from build123d import *

# Parameters (mm, degrees)
SKETCH_1_W          = 80
SKETCH_1_H          = 80
EXTRUDE_1_DEPTH     = 2
CUT_EXTRUDE_1_DEPTH = 10


with BuildPart() as part:
    # ｽｹｯﾁ1 → ﾎﾞｽ - 押し出し1 (new body)
    with BuildSketch(Plane.XY):
        Rectangle(SKETCH_1_W, SKETCH_1_H)
    extrude(amount=EXTRUDE_1_DEPTH)

    # ｽｹｯﾁ2 → ｶｯﾄ - 押し出し1 (cut)
    with BuildSketch(Plane.XY.offset(2)):
        with BuildLine():
            ThreePointArc((29.5, -25), (26.318019485, -26.318019485), (25, -29.5))
            Line((25, -29.5), (29.5, -29.5))
            Line((29.5, -29.5), (29.5, -25))
        make_face()
        with BuildLine():
            Line((29.5, -29.5), (25, -29.5))
            ThreePointArc((25, -29.5), (29.5, -34), (34, -29.5))
            ThreePointArc((34, -29.5), (32.681980515, -26.318019485), (29.5, -25))
            Line((29.5, -25), (29.5, -29.5))
        make_face()
        with BuildLine():
            ThreePointArc((21.99, -17.49), (18.808019485, -18.808019485), (17.49, -21.99))
            Line((17.49, -21.99), (21.99, -21.99))
            Line((21.99, -21.99), (21.99, -17.49))
        make_face()
        with BuildLine():
            Line((21.99, -21.99), (17.49, -21.99))
            ThreePointArc((17.49, -21.99), (21.99, -26.49), (26.49, -21.99))
            ThreePointArc((26.49, -21.99), (25.171980515, -18.808019485), (21.99, -17.49))
            Line((21.99, -17.49), (21.99, -21.99))
        make_face()
        with BuildLine():
            ThreePointArc((25, 29.5), (26.318019485, 26.318019485), (29.5, 25))
            Line((29.5, 25), (29.5, 29.5))
            Line((29.5, 29.5), (25, 29.5))
        make_face()
        with BuildLine():
            Line((29.5, 29.5), (29.5, 25))
            ThreePointArc((29.5, 25), (32.681980515, 26.318019485), (34, 29.5))
            ThreePointArc((34, 29.5), (29.5, 34), (25, 29.5))
            Line((25, 29.5), (29.5, 29.5))
        make_face()
        with BuildLine():
            ThreePointArc((17.49, 21.99), (18.808019485, 18.808019485), (21.99, 17.49))
            Line((21.99, 17.49), (21.99, 21.99))
            Line((21.99, 21.99), (17.49, 21.99))
        make_face()
        with BuildLine():
            Line((21.99, 21.99), (21.99, 17.49))
            ThreePointArc((21.99, 17.49), (25.171980515, 18.808019485), (26.49, 21.99))
            ThreePointArc((26.49, 21.99), (21.99, 26.49), (17.49, 21.99))
            Line((17.49, 21.99), (21.99, 21.99))
        make_face()
        with BuildLine():
            ThreePointArc((-21.99, -17.49), (-25.171980515, -25.171980515), (-17.49, -21.99))
            Line((-17.49, -21.99), (-21.99, -21.99))
            Line((-21.99, -21.99), (-21.99, -17.49))
        make_face()
        with BuildLine():
            Line((-21.99, -21.99), (-17.49, -21.99))
            ThreePointArc((-17.49, -21.99), (-18.808019485, -18.808019485), (-21.99, -17.49))
            Line((-21.99, -17.49), (-21.99, -21.99))
        make_face()
        with BuildLine():
            ThreePointArc((-29.5, -25), (-32.681980515, -32.681980515), (-25, -29.5))
            Line((-25, -29.5), (-29.5, -29.5))
            Line((-29.5, -29.5), (-29.5, -25))
        make_face()
        with BuildLine():
            Line((-29.5, -29.5), (-25, -29.5))
            ThreePointArc((-25, -29.5), (-26.318019485, -26.318019485), (-29.5, -25))
            Line((-29.5, -25), (-29.5, -29.5))
        make_face()
        with BuildLine():
            ThreePointArc((-17.49, 21.99), (-25.171980515, 25.171980515), (-21.99, 17.49))
            Line((-21.99, 17.49), (-21.99, 21.99))
            Line((-21.99, 21.99), (-17.49, 21.99))
        make_face()
        with BuildLine():
            Line((-21.99, 21.99), (-21.99, 17.49))
            ThreePointArc((-21.99, 17.49), (-18.808019485, 18.808019485), (-17.49, 21.99))
            Line((-17.49, 21.99), (-21.99, 21.99))
        make_face()
        with BuildLine():
            ThreePointArc((-25, 29.5), (-32.681980515, 32.681980515), (-29.5, 25))
            Line((-29.5, 25), (-29.5, 29.5))
            Line((-29.5, 29.5), (-25, 29.5))
        make_face()
        with BuildLine():
            Line((-29.5, 29.5), (-29.5, 25))
            ThreePointArc((-29.5, 25), (-26.318019485, 26.318019485), (-25, 29.5))
            Line((-25, 29.5), (-29.5, 29.5))
        make_face()
    extrude(amount=-CUT_EXTRUDE_1_DEPTH, mode=Mode.SUBTRACT)


solid = part.part
Geometry check sheet. Reference: the model listing, model coordinates, mm. Round coordinates to 2 decimals unless told otherwise and drop trailing zeros. Order: outer loops, then holes, each group sorted by start corner. A loop starts at its lowest first (then second) coordinate and runs counter-clockwise, first axis right, second up. Notation, with made-up numbers: M -23,-31 L 19,-31 A7 cw 19,-26 Z; hole C -16,-5 d3. An arc over 180 degrees is marked long. Answer in a Markdown table with one row per item. Add a question column.
Item 1: Sectioned sample at A-A, the plane z = 0.5. State how many separate pieces and enclosed holes the cut face has, plus the area to 3 significant figures.
Item 2: Material ranges on L1, parallel to X at y = 21.99, z = 1.3; L2, parallel to X at y = -29.5, z = 1.2, recorded low to high. Write a range as [from, to].
Item 3: Sectioned sample at B-B, the plane x = -31. Enter the section's corners in (y, z).
Item 4: Depth check by flat-ended pin: pin 1 Ø5.5 at (x, y) = (-29.5, -29.5) entering from -Z. Enter the tip coordinate at first touch or a pass-through.
Filled in:
| question | item | result |
|---|---|---|
| 1 | separate pieces | 1 |
| 1 | enclosed holes | 8 |
| 1 | area | 5,890 mm² |
| 2 | L1 | x = [-40, -26.49], [-17.49, 17.49], [26.49, 40] |
| 2 | L2 | x = [-40, -34], [-25, 25], [34, 40] |
| 3 | outline | M -40,0 L -33.74,0 L -33.74,2 L -40,2 Z; M -25.26,0 L 25.26,0 L 25.26,2 L -25.26,2 Z; M 33.74,0 L 40,0 L 40,2 L 33.74,2 Z |
| 4 | pin 1 | passes through |
